Verification items for the finished model (mm, model axes). A direction names the side the tool comes from. Round coordinates to 2 decimals unless told otherwise and drop trailing zeros. Loops run counter-clockwise (first coordinate to the right, second up) from the corner with the lowest first, then second, coordinate; pieces in that order, holes last. Notation, with made-up numbers: M 55,2 L 95,2 A34 cw 95,37 Z; hole C -22.5,27.25 d4. An arc over 180 degrees is marked long. One line per item, written item: value.
Autodesk Inventor part; units mm, degrees
ref_plane "YZ Plane" through (0, 0, 0) normal (1, 0, 0) x (0, 1, 0)
ref_plane "XZ Plane" through (0, 0, 0) normal (0, 1, 0) x (-1, 0, 0)
ref_plane "XY Plane" through (0, 0, 0) normal (0, 0, 1) x (1, 0, 0)
sketch "Sketch1" plane through (0, 0, 0) normal (0, 0, 1) x (1, 0, 0)
  line L0 (0, 0) -> (40, 0)
  line L1 (40, 0) -> (40, 4)
  line L2 (0, 4) -> (40, 4) construction
  line L3 (0, 0) -> (0, 4)
  line L4 (120, 0) -> (160, 0)
  line L5 (160, 0) -> (160, 4)
  line L6 (120, 4) -> (160, 4) construction
  line L7 (120, 0) -> (120, 4)
  line L8 (0, 4) -> (0, 26.1116)
  line L9 (0, 26.1116) -> (160, 54.3239)
  line L10 (160, 54.3239) -> (160, 4)
  line L11 (120, 4) -> (101.5, 4)
  line L12 (61.5, 4) -> (61.5, 0) construction
  line L13 (58.5, 4) -> (58.5, 0) construction
  line L14 (98.5, 4) -> (98.5, 0) construction
  line L15 (101.5, 4) -> (101.5, 0) construction
  line L16 (58.5, 4) -> (61.5, 4) construction
  line L17 (61.5, 4) -> (61.5, 16)
  line L18 (61.5, 16) -> (58.5, 16)
  line L19 (58.5, 16) -> (58.5, 4)
  line L20 (57.3, 8.8) -> (62.7, 8.8)
  line L21 (62.7, 8.8) -> (62.7, 11.2)
  line L22 (62.7, 11.2) -> (57.3, 11.2)
  line L23 (57.3, 11.2) -> (57.3, 8.8)
  line L24 (98.5, 4) -> (101.5, 4) construction
  line L25 (101.5, 4) -> (101.5, 16)
  line L26 (101.5, 16) -> (98.5, 16)
  line L27 (98.5, 16) -> (98.5, 4)
  line L28 (102.7, 8.8) -> (97.3, 8.8)
  line L29 (97.3, 8.8) -> (97.3, 11.2)
  line L30 (97.3, 11.2) -> (102.7, 11.2)
  line L31 (102.7, 11.2) -> (102.7, 8.8)
  line L32 (58.5, 4) -> (40, 4)
  line L33 (61.5, 4) -> (58.5, 4)
  line L34 (98.5, 4) -> (61.5, 4)
  line L35 (101.5, 4) -> (98.5, 4)
  line L36 (11.5846, 18) -> (50.9769, 24.9459)
  line L37 (50.9769, 24.9459) -> (50.2823, 28.8852)
  line L38 (50.2823, 28.8852) -> (10.89, 21.9392)
  line L39 (10.89, 21.9392) -> (11.5846, 18)
  line L40 (110.7596, 39.5489) -> (150.1519, 46.4949)
  line L41 (150.1519, 46.4949) -> (150.8465, 42.5556)
  line L42 (150.8465, 42.5556) -> (111.4542, 35.6097)
  line L43 (111.4542, 35.6097) -> (110.7596, 39.5489)
  line L44 (150.1519, 46.4949) -> (160, 48.2314) construction
  line L45 (50.6296, 26.9155) -> (65.7489, 29.5815) construction
  line L46 (65.7489, 29.5815) -> (80.8682, 32.2474) construction
  line L47 (80.8682, 32.2474) -> (95.9876, 34.9134) construction
  line L48 (95.9876, 34.9134) -> (111.1069, 37.5793) construction
  circle A0 centre (65.7489, 29.5815) radius 1.5
  circle A1 centre (95.9876, 34.9134) radius 1.5
  point P0 (60, 11.2)
  point P1 (60, 16)
  point P2 (62.7, 10)
  point P3 (61.5, 10)
  point P4 (100, 11.2)
  point P5 (100, 16)
  point P6 (58.5, 8.8)
  point P7 (58.5, 11.2)
  point P8 (61.5, 11.2)
  point P9 (61.5, 8.8)
  point P10 (98.5, 8.8)
  point P11 (98.5, 11.2)
  point P12 (101.5, 11.2)
  point P13 (101.5, 8.8)
  dimension "d0" = 3
  dimension "d1" = 12
  dimension "d2" = 5.4
  dimension "d3" = 2.4
  dimension "d4" = 10
  dimension "d6" = 40
  dimension "d7" = 3
  dimension "d9" = 4
  dimension "d10" = 14
  dimension "d11" = 6
  dimension "d12" = 10
  dimension "d13" = 10
extrude "Extrusion1" add sketch "Sketch1" along normal blind 4 contours L3 L8 L9 L10 L5 L4 L7 L11 L25 L28 L31 L30 L26 L27 L29 L34 L17 L20 L21 L22 L18 L19 L23 L32 L1 L0
fillet "Fillet1" radius 12 1 edges at (160, 54.3239, 2)
fillet "Fillet2" radius 5 1 edges at (0, 26.1116, 2)
properties part number "Pannel_Side" material "MDF Medium Density Fiberboard"
(1) Depth check by flat-ended pin: pin 1 Ø0.6 at (x, z) = (58, 2) entering from +Y; pin 2 Ø2 at (x, z) = (48, 2) entering from -Y. Enter the tip coordinate at first touch or a pass-through.
Completed:
pin 1: stops at y = 36.39
pin 2: stops at y = 4
(2) Sectioned sample at A-A on y = 6. Enter the section's corners in (x, z), and give its area (3 significant figures).
Completed:
outline: M 0,0 L 58.5,0 L 58.5,4 L 0,4 Z; M 61.5,0 L 98.5,0 L 98.5,4 L 61.5,4 Z; M 101.5,0 L 160,0 L 160,4 L 101.5,4 Z
area: 616 mm^2
(3) Tool access check on faces 5 (the face through (150.494, 44.553, 1.972)), 6 (the face through (140, 0, 2)), 7 (the face through (61.5, 14, 2)). Record the directions out of +Z, -Z, +X, -X, +Y, -Y that give a thin tool (end or side, any length) a straight path to the whole face; none if there is none.
Completed:
face 5: +Z, -Z
face 6: +Z, -Z, +X, -X, -Y
face 7: +Z, -Z, -Y
(4) Sectioned sample at D-D on x = 71. Enter the section's corners in (y, z), and give its area (3 significant figures).
Completed:
outline: M 4,0 L 38.63,0 L 38.63,4 L 4,4 Z
area: 139 mm^2
(5) Mould release check, pull along Y, two halves, no side actions. Record for faces 1 (the face through (74.032, 39.165, 1.972)), 2 (the face through (97, 21, 4)), 3 (the face through (11.23, 20, 1.97)), 4 (the face through (31.005, 21.424, 1.972)): +Y half, -Y half, draft (parallel to the pull), parting line (faces both ways), or undercut.
Completed:
face 1: +Y half
face 2: draft
face 3: undercut
face 4: undercut
(6) Thickness scan on L1, parallel to X at y = 9, z = 1.3; L2, parallel to X at y = 14, z = 1.5; L3, parallel to Y at x = 43, z = 0.7. Record the ranges inside material, lowest first. Write a range as from..to.
Completed:
L1: x = 0..57.3, 62.7..97.3, 102.7..160
L2: x = 0..58.5, 61.5..98.5, 101.5..160
L3: y = 4..23.54, 27.6..33.69
(7) Sectioned sample at B-B on x = 122. Enter the section's corners in (y, z).
Completed:
outline: M 0,0 L 37.47,0 L 37.47,4 L 0,4 Z; M 41.53,0 L 47.62,0 L 47.62,4 L 41.53,4 Z
(8) Sectioned sample at C-C on y = 20. Enter the section's corners in (x, z), and give its area (3 significant figures).
Completed:
outline: M 0,0 L 11.23,0 L 11.23,4 L 0,4 Z; M 22.93,0 L 160,0 L 160,4 L 22.93,4 Z
area: 593 mm^2
